Check sheet for the drawn part. Datum: minimum x, y, z corner. Units: mm. A direction names the side the tool comes from. Give positions to 0.01 mm unless a question says otherwise; leave off trailing zeros. Write each loop counter-clockwise with the first axis right and the second up, starting at its lowest first coordinate (ties: lowest second). Pieces come first, ordered by that corner, then holes.
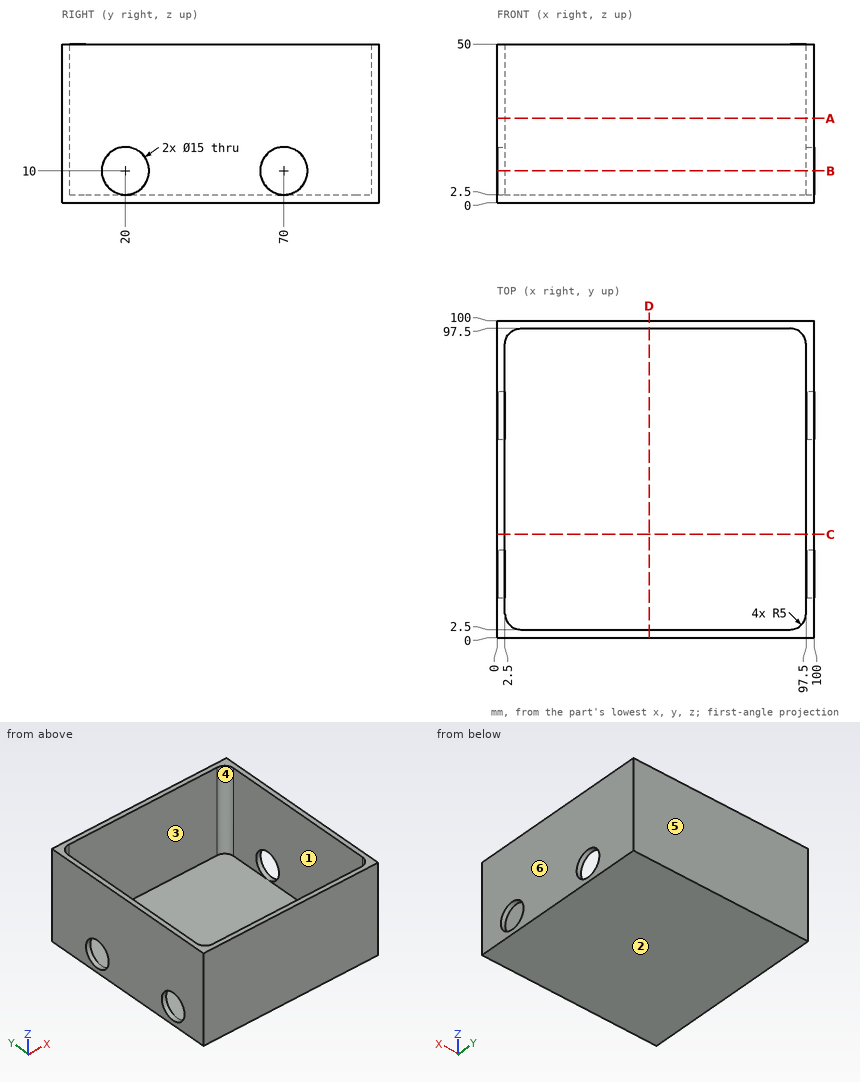
1) Gauge pin test, flat end, axial feed: pin 1 (1.5 mm diameter, centred on x = 64.5, y = 89, fed in from +Z). Record the tip position at first contact, or that the pin passes through.
2) Sectioned sample at A-A on z = 26.5. Record the boundary of the cut face in (x, y), then the cut area to 3 significant figures.
3) Sectioned sample at C-C on y = 32.5. Record the boundary of the cut face in (x, z).
4) Draft check along Y on the marked faces 3, 4, 5 and 6. Enter one of: +Y half, -Y half, draft (parallel to the pull), parting line (faces both ways), or undercut.
5) Scan lines: L1, parallel to Y at x = 98.3, z = 10; L2, parallel to Z at x = 98, y = 20; L3, parallel to X at y = 67.5, z = 23. Record each from-to range of solid material in increasing order.
6) Sectioned sample at B-B on z = 10. Record the boundary of the cut face in (x, y), then the cut area to 3 significant figures.
7) Access from +Z, -Z, +X, -X, +Y, -Y to the whole of each face (thin tool, end or side, straight path). Record for the marked faces 1 and 2.
Answers below:
1. pin 1: stops at z = 2.5
2. outline: (0, 0) - (100, 0) - (100, 100) - (0, 100) - close; hole (2.5, 7.5) arc R5 ccw to (7.5, 2.5) - (92.5, 2.5) arc R5 ccw to (97.5, 7.5) - (97.5, 92.5) arc R5 ccw to (92.5, 97.5) - (7.5, 97.5) arc R5 ccw to (2.5, 92.5) - close
2. area: 996 mm2
3. outline: (0, 0) - (100, 0) - (100, 50) - (97.5, 50) - (97.5, 2.5) - (2.5, 2.5) - (2.5, 50) - (0, 50) - close
4. face 3: undercut
4. face 4: undercut
4. face 5: +Y half
4. face 6: draft
5. L1: y = 0 to 12.5, 27.5 to 62.5, 77.5 to 100
5. L2: z = 0 to 2.5, 17.5 to 50
5. L3: x = 0 to 2.5, 97.5 to 100
6. outline: (0, 0) - (100, 0) - (100, 12.5) - (97.5, 12.5) - (97.5, 7.5) arc R5 cw to (92.5, 2.5) - (7.5, 2.5) arc R5 cw to (2.5, 7.5) - (2.5, 12.5) - (0, 12.5) - close; (0, 27.5) - (2.5, 27.5) - (2.5, 62.5) - (0, 62.5) - close; (0, 77.5) - (2.5, 77.5) - (2.5, 92.5) arc R5 cw to (7.5, 97.5) - (92.5, 97.5) arc R5 cw to (97.5, 92.5) - (97.5, 77.5) - (100, 77.5) - (100, 100) - (0, 100) - close; (97.5, 27.5) - (100, 27.5) - (100, 62.5) - (97.5, 62.5) - close
6. area: 846 mm2
7. face 1: +Z
7. face 2: -Z, +X, -X, +Y, -Y
